Autodesk Inventor part; units mm, degrees
ref_plane "YZ Plane" through (0, 0, 0) normal (1, 0, 0) x (0, 1, 0)
ref_plane "XZ Plane" through (0, 0, 0) normal (0, 1, 0) x (-1, 0, 0)
ref_plane "XY Plane" through (0, 0, 0) normal (0, 0, 1) x (1, 0, 0)
sketch "Sketch1" plane through (0, 0, 0) normal (0, 1, 0) x (-1, 0, 0)
  circle A0 centre (0, 0) radius 2
  line L0 (-18.4961, 38.8165) -> (-18.4961, -38.8135)
  line L1 (18.4961, 38.8135) -> (-18.4961, -38.8135) construction
  line L2 (-18.4961, 38.8165) -> (18.4961, -38.8165) construction
  circle A1 centre (0, 31) radius 5
  circle A2 centre (0, -31) radius 5
  arc A3 (18.5039, 38.815) -> (-18.4961, 38.8188) centre (0, 0) ccw
  arc A4 (-18.4961, -38.8188) -> (18.5039, -38.815) centre (0, 0) ccw
  line L3 (18.5039, 38.815) -> (18.5039, -38.815)
  line L4 (-18.4961, -38.8135) -> (-18.4961, -38.8188)
  line L5 (-18.4961, 38.8165) -> (-18.4961, 38.8188)
  dimension "d0" = 2
  dimension "d4" = 10
  dimension "d5" = 10
  dimension "d6" = 31
  dimension "d7" = 31
  dimension "d8" = 77.63
  dimension "d9" = 37
  dimension "d10" = 43
  dimension "d11" = 43
  dimension "d12" = 77.63
extrude "Extrusion1" add sketch "Sketch1" along normal blind 10
sketch "Sketch2" plane through (18.4961, 0, 38.8188) normal (1, 0, 0) x (0, 0, -1)
  line L0 (0, 0) -> (77.6375, 0)
  line L1 (0, 10) -> (77.6375, 10)
  line L2 (0.0038, 0) -> (-4.1812, 0)
  line L3 (-4.1812, 0) -> (16.8188, 0)
  line L4 (16.8188, 0) -> (16.8188, -13)
  line L5 (16.8188, -13) -> (20.7888, -13)
  line L6 (81.8188, 0) -> (77.6338, 0)
  line L7 (81.8188, 0) -> (60.8188, 0)
  line L8 (60.8188, 0) -> (60.8188, -13)
  line L9 (60.8188, -13) -> (56.8488, -13)
  arc A0 (56.8488, -13) -> (20.7888, -13) centre (38.8188, -19.0031) ccw
  arc A1 (63.4021, 10) -> (14.2354, 10) centre (38.8188, -19.0031) ccw
  line L10 (36.8188, 10) -> (40.8188, 10)
  point P0 (38.8188, 0)
  point P1 (38.8188, 19.0169)
  dimension "d15" = 21
  dimension "d16" = 13
  dimension "d17" = 3.97
  dimension "d18" = 21
  dimension "d19" = 13
  dimension "d20" = 3.97
  dimension "d22" = 38.02
extrude "Extrusion2" add sketch "Sketch2" against normal blind 37
sketch "Sketch3" plane through (0, 10, 0) normal (0, -1, 0) x (1, 0, 0)
  circle A0 centre (0, 0) radius 2
extrude "Extrusion3" cut sketch "Sketch3" along normal through all both and the other way through all
sketch "Sketch4" plane through (0, 0, 0) normal (0, -1, 0) x (1, 0, 0)
  circle A0 centre (0, 31) radius 5
  arc A1 (-12, 31) -> (12, 31) centre (0, 31) ccw
  circle A2 centre (0, 31) radius 10.5
  arc A3 (-10.5, 31) -> (10.5, 31) centre (0, 31) ccw
  line L0 (12, 31) -> (-12, 31)
  point P0 (10.5, 31)
  dimension "d27" = 12
extrude "Extrusion4" cut sketch "Sketch4" against normal blind 3.032 from surface at -10 contours L0 A1 A2
sketch "Sketch5" plane through (0, 10, 0) normal (0, 1, 0) x (1, 0, 0)
  line L0 (-18.5039, 24.5833) -> (18.4961, 24.5833)
  circle A0 centre (0, 31) radius 5
  circle A1 centre (0, 31) radius 10.5
  arc A2 (-12, 31) -> (12, 31) centre (0, 31) ccw
  arc A3 (-10.5, 31) -> (10.5, 31) centre (0, 31) ccw
  line L1 (12, 31) -> (-12, 31)
  point P0 (8.3112, 24.5833)
  point P1 (-8.3112, 24.5833)
  dimension "d30" = 12
extrude "Extrusion5" cut sketch "Sketch5" along normal through all contours A2 L1 A1 L0 | L0 A1 A2 | L0 A1 | L0 A1 L1 A2
sketch "Sketch6" plane through (0, 13.032, 31) normal (0, -1, 0) x (1, 0, 0)
  arc A0 (-5.7661, -10.5239) -> (5.7661, -10.5239) centre (0, 0) ccw
  line L0 (-5.7661, -10.5239) -> (5.7661, -10.5239)
  spline S0 degree 6 poles (8.3112, -6.4167) (8.1303, -6.651) (7.9395, -6.8817) (7.739, -7.108) (7.5289, -7.3291) (7.3096, -7.5442) (6.6527, -8.1442) (6.1935, -8.5115) (5.7064, -8.85) (5.1948, -9.156) (4.663, -9.4266) (3.9079, -9.7483) (3.6976, -9.8316) (3.4851, -9.9094) (3.2708, -9.9817) (3.0547, -10.0484) (2.3754, -10.239) (1.9069, -10.3432) (1.4335, -10.4215) (0.9567, -10.4739) (0.4783, -10.5) (-0.4841, -10.5) (-0.9683, -10.4732) (-1.4508, -10.4196) (-1.9299, -10.3394) (-2.4038, -10.2327) (-3.0854, -10.0389) (-3.2986, -9.9724) (-3.5101, -9.9004) (-3.7198, -9.8231) (-3.9273, -9.7404) (-4.6765, -9.4197) (-5.2053, -9.1498) (-5.7139, -8.8448) (-6.1983, -8.5077) (-6.655, -8.1422) (-7.3097, -7.5441) (-7.529, -7.3291) (-7.739, -7.108) (-7.9396, -6.8817) (-8.1303, -6.6509) (-8.3112, -6.4167) knots 0 0 0 0 0 0 0 0.097765 0.097765 0.097765 0.097765 0.097765 0.281656 0.281656 0.281656 0.281656 0.281656 0.351588 0.351588 0.351588 0.351588 0.351588 0.499999 0.499999 0.499999 0.499999 0.499999 0.65021 0.65021 0.65021 0.65021 0.65021 0.719277 0.719277 0.719277 0.719277 0.719277 0.902242 0.902242 0.902242 0.902242 0.902242 1 1 1 1 1 1 1
  line L1 (8.3112, -6.4167) -> (-8.3112, -6.4167)
  point P0 (0, -31)
extrude "Extrusion6" cut sketch "Sketch6" against normal blind 10 from surface at 3.032
properties part number "cap" material "Brass, Soft Yellow"
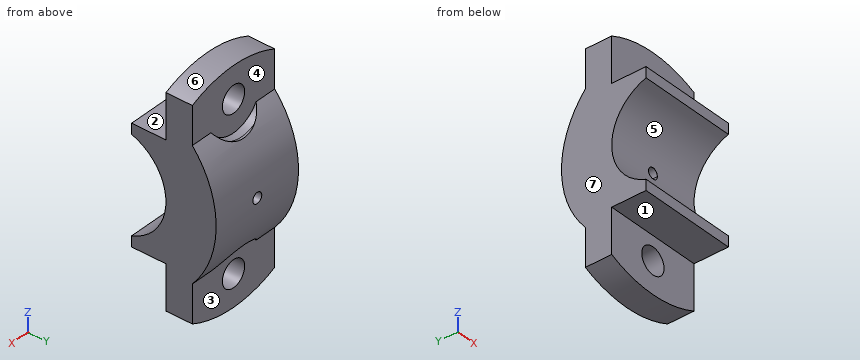
Source: CAD feature listing. Evaluate the final solid. Frame: model axes, mm. Face numbers are marked on the shaded views. A direction names the side the tool comes from. Coordinates: 2 decimals unless noted, no trailing zeros. Write each loop counter-clockwise with the first axis right and the second up, starting at its lowest first coordinate (ties: lowest second). Pieces come first, ordered by that corner, then holes. Notation, with made-up numbers: M -3.5,8 L 10.5,8 A14 ccw 10.5,24 Z; hole C -38,-23.5 d7. An arc over 180 degrees is marked long. Answer as a JSON object with one key per item and string values.
1. Cut plane D-D on y = -4. Output: boundary loops of the cut face in (x, z), plus the area to 3 significant figures.
Evaluation:
{"outline": "M -18.5,-22 L 18.5,-22 L 18.5,-11.66 L -18.5,-11.66 Z; M -18.5,11.66 L 18.5,11.66 L 18.5,22 L -18.5,22 Z", "area": "765 mm^2"}
2. Access query for the marked faces 1, 2, 3 and 4. Directions: +Z, -Z, +X, -X, +Y, -Y. A direction counts if a zero-diameter tool reaches every point of the face in a straight line with its end or side. Return the directions, or none.
Evaluation:
{"face 1": "-Z, +X, -X, -Y", "face 2": "+Z, +X, -X, -Y", "face 3": "-Z, +Y", "face 4": "+Z, +Y"}
3. Draft query along Z for the marked faces 5, 6 and 7. Return one class per face: released by +Z, released by -Z, zero draft, split by the parting line, or undercut.
Evaluation:
{"face 5": "undercut", "face 6": "released by +Z", "face 7": "zero draft"}
4. Cut plane A-A on y = 5. Output: boundary loops of the cut face in (x, z) (3 decimals).
Evaluation:
{"outline": "M -18.504,-38.815 A43 ccw 18.496,-38.819 L 18.496,38.819 A43 ccw -18.504,38.815 Z; hole C 0,-31 d10; hole C 0,31 d10; hole C 0,0 d4"}
5. Cut plane C-C on x = 0. Output: boundary loops of the cut face in (y, z), plus the area to 3 significant figures.
Evaluation:
{"outline": "M -13,-22 L 0,-22 L 0,-26 L 10,-26 L 10,-19 L 13.93,-19 A38.02 ccw 18.96,-2 L -0.11,-2 A19 cw -13,-18.03 Z; M -13,18.03 A19 cw -0.11,2 L 18.96,2 A38.02 ccw 13.93,19 L 10,19 L 10,26 L 0,26 L 0,22 L -13,22 Z; M 0,-43 L 10,-43 L 10,-36 L 0,-36 Z; M 0,36 L 10,36 L 10,43 L 0,43 Z", "area": "1,090 mm^2"}
6. Ray query, L1, parallel to Z at x = 0, y = 8; L2, parallel to Z at x = 3, y = 0.5; L3, parallel to X at y = 15.5, z = 0. Return the intervals inside material, ascending.
Evaluation:
{"L1": "-43 to -36, -26 to -2, 2 to 26, 36 to 43", "L2": "-42.9 to -35, -27 to 27, 35 to 42.9", "L3": "-18.5 to -2, 2 to 18.5"}
7. Contact query for flat-ended pins moving along their axis: P1, Ø19, axis at x = 5, z = 29.5, coming from the +Y side; P2, Ø17, axis at x = -4.5, z = 35.5, coming from the -Y side; P3, Ø6, axis at x = -2.5, y = -2, coming from the -Z side; P4, Ø6, axis at y = 14, z = -34, coming from the -X side. Output: stop coordinate, or through.
Evaluation:
{"P1": "y = 13.33", "P2": "y = 0", "P3": "z = -43", "P4": "through"}
8. Cut plane B-B on z = 31. Output: boundary loops of the cut face in (x, y).
Evaluation:
{"outline": "M -18.5,0 L -5,0 L -5,10 L -18.5,10 Z; M 5,0 L 18.5,0 L 18.5,10 L 5,10 Z"}
